from build123d import *

# Parameters (mm, degrees)
F0_R     = 2.413
F1_DEPTH = 6.35
F2_SIZE  = 1.9812


with BuildPart() as f1:
    # F0 (on Top) → F1 (new body)
    with BuildSketch(Plane.XY):
        with BuildLine():
            ThreePointArc((-72.451897, -44.454429), (-70.592025, -48.944557), (-66.101897, -50.804429))
            Line((-66.101897, -50.804429), (73.598103, -50.804429))
            ThreePointArc((73.598103, -50.804429), (78.088231, -48.944557), (79.948103, -44.454429))
            Line((79.948103, -44.454429), (79.948103, 44.445571))
            ThreePointArc((79.948103, 44.445571), (78.088231, 48.935699), (73.598103, 50.795571))
            Line((73.598103, 50.795571), (-66.101897, 50.795571))
            ThreePointArc((-66.101897, 50.795571), (-70.592025, 48.935699), (-72.451897, 44.445571))
            Line((-72.451897, 44.445571), (-72.451897, -44.454429))
        make_face()
        with Locations((-66.101897, -44.454429)):
            Circle(F0_R, mode=Mode.SUBTRACT)
        with Locations((73.598103, -44.454429)):
            Circle(F0_R, mode=Mode.SUBTRACT)
        with BuildLine():
            ThreePointArc((10.928676, -2.263215), (12.523538, -0.683077), (14.103676, -2.27794))
            Line((14.103676, -2.27794), (14.103676, -24.50294))
            ThreePointArc((14.103676, -24.50294), (12.508813, -26.083077), (10.928676, -24.488215))
            Line((10.928676, -24.488215), (10.928676, -2.263215))
        make_face(mode=Mode.SUBTRACT)
        with BuildLine():
            ThreePointArc((-28.991299, 11.1125), (-27.403799, 12.7), (-25.816299, 11.1125))
            Line((-25.816299, 11.1125), (-25.816299, -11.1125))
            ThreePointArc((-25.816299, -11.1125), (-27.403799, -12.7), (-28.991299, -11.1125))
            Line((-28.991299, -11.1125), (-28.991299, 11.1125))
        make_face(mode=Mode.SUBTRACT)
        with BuildLine():
            ThreePointArc((-25.986542, 26.997524), (-25.754058, 27.55879), (-25.192792, 27.791274))
            Line((-25.192792, 27.791274), (25.607208, 27.791274))
            ThreePointArc((25.607208, 27.791274), (26.168474, 27.55879), (26.400958, 26.997524))
            Line((26.400958, 26.997524), (26.400958, 21.981024))
            ThreePointArc((26.400958, 21.981024), (26.168474, 21.419758), (25.607208, 21.187274))
            Line((25.607208, 21.187274), (-25.192792, 21.187274))
            ThreePointArc((-25.192792, 21.187274), (-25.754058, 21.419758), (-25.986542, 21.981024))
            Line((-25.986542, 21.981024), (-25.986542, 26.997524))
        make_face(mode=Mode.SUBTRACT)
        with Locations((-66.101897, 44.445571)):
            Circle(F0_R, mode=Mode.SUBTRACT)
        with Locations((73.598103, 44.445571)):
            Circle(F0_R, mode=Mode.SUBTRACT)
    extrude(amount=F1_DEPTH)

    # F2
    f2_edges = [f1.edges().sort_by_distance(p)[0] for p in [
        (-68.514897, -44.454429, 6.35),
        (71.185103, -44.454429, 6.35),
        (71.185103, 44.445571, 6.35),
        (-68.514897, 44.445571, 6.35),
    ]]
    chamfer(f2_edges, length=F2_SIZE)


solid = f1.part
Geometry: final body of the model. Coordinates: model frame, mm. A direction names the side the tool comes from. Give positions to 0.01 mm unless a question says otherwise; leave off trailing zeros. Loops run counter-clockwise (first coordinate to the right, second up) from the corner with the lowest first, then second, coordinate; pieces in that order, holes last. Notation, with made-up numbers: (42, 63) - (55, 63) arc R27 ccw to (55, 97) - close; hole circle Ø4 at (87.5, 3.5). An arc over 180 degrees is marked (long way). Answer as CSV lines item,"result". Start each with the question number.
1. Draft query along X for faces 3 (the face through (-72.452, 1, 3)), 4 (the face through (26.401, 25, 3)), 5 (the face through (3, 1, 6.35)). Return one class per face: released by +X, released by -X, zero draft, split by the parting line, or undercut.
2. Section D-D, the plane y = 4.5. Return loops of the section in (x, z).
3. Section A-A, the plane y = -9.5. Return loops of the section in (x, z), plus the area to 3 significant figures.
4. Pin query (flat end, axial travel): P1, Ø3, axis at x = 73.6, y = -44.45, coming from the -Z side; P2, Ø5.5, axis at x = -66.1, y = 44.45, coming from the +Z side. Return the tip coordinate at first contact, or that it passes through.
5. Section C-C, the plane z = 1.75. Give the number of separate pieces and of enclosed holes in the cut face, plus the area to 3 significant figures.
6. Ray query, L1, parallel to X at y = -4, z = 3; L2, parallel to X at y = 7, z = 2; L3, parallel to X at y = 23.5, z = 4.5. Return the intervals inside material, ascending.
7. Section B-B, the plane x = -22.5. Return loops of the section in (y, z).
8. Reachability of faces 1 (the face through (-25.816, 0, 3)), 2 (the face through (78.04, -48.99, 3.13)) from +Z, -Z, +X, -X, +Y, -Y: full face, straight path, thin tool, end or side. Return the list, or none.
Answers:
1,face 3,"released by -X"
1,face 4,"undercut"
1,face 5,"zero draft"
2,outline,"(-72.45, 0) - (-28.99, 0) - (-28.99, 6.35) - (-72.45, 6.35) - close; (-25.82, 0) - (79.95, 0) - (79.95, 6.35) - (-25.82, 6.35) - close"
3,outline,"(-72.45, 0) - (-28.99, 0) - (-28.99, 6.35) - (-72.45, 6.35) - close; (-25.82, 0) - (10.93, 0) - (10.93, 6.35) - (-25.82, 6.35) - close; (14.1, 0) - (79.95, 0) - (79.95, 6.35) - (14.1, 6.35) - close"
3,area,"927 mm2"
4,P1,"passes through"
4,P2,"stops at z = 4.71"
5,separate pieces,"1"
5,enclosed holes,"7"
5,area,"14,900 mm2"
6,L1,"x = -72.45 to -28.99, -25.82 to 10.93, 14.1 to 79.95"
6,L2,"x = -72.45 to -28.99, -25.82 to 79.95"
6,L3,"x = -72.45 to -25.99, 26.4 to 79.95"
7,outline,"(-50.8, 0) - (21.19, 0) - (21.19, 6.35) - (-50.8, 6.35) - close; (27.79, 0) - (50.8, 0) - (50.8, 6.35) - (27.79, 6.35) - close"
8,face 1,"+Z, -Z"
8,face 2,"+Z, -Z, +X, -Y"
